from build123d import *

# Parameters (mm, degrees)
SKETCH090_R             = 5
SKETCH090_R_2           = 2.25
PAD032_DEPTH            = 2
SKETCH091_R             = 5
SKETCH091_R_2           = 3.75
PAD033_DEPTH            = 4
BODY011_PLACEMENT_ANGLE = 90


with BuildPart() as part:
    # Sketch090 → Pad032 (new body)
    with BuildSketch(Plane.XZ):
        Circle(SKETCH090_R)
        Circle(SKETCH090_R_2, mode=Mode.SUBTRACT)
    extrude(amount=PAD032_DEPTH)

    # Sketch091 (on Face4 of Pad032) → Pad033 (join)
    with BuildSketch(Plane.XZ.offset(2)):
        Circle(SKETCH091_R)
        Circle(SKETCH091_R_2, mode=Mode.SUBTRACT)
    extrude(amount=PAD033_DEPTH)


with BuildPart() as part_1:
    # Body011 placement: moved
    add(part.part.moved(Location((62, 89, 34))).rotate(Axis((62, 89, 34), (-1, 0, 0)), BODY011_PLACEMENT_ANGLE))


solid = part_1.part
Source: CAD feature listing. Evaluate the final solid. Frame: model axes, mm. A direction names the side the tool comes from. Round coordinates to 2 decimals unless told otherwise and drop trailing zeros. Loops run counter-clockwise (first coordinate to the right, second up) from the corner with the lowest first, then second, coordinate; pieces in that order, holes last.
Q1. First-contact query: P1, Ø2, axis at y = 87, z = 38.5, coming from the +X side; P2, Ø3, axis at x = 65, z = 36.5, coming from the -Y side; P3, Ø1, axis at y = 90, z = 37, coming from the +X side. Flat tips, straight axial feed; report the tip coordinate or a pass-through.
Q2. Section C-C, the plane y = 92. Return loops of the section in (x, z).
Q3. Mould query, pull axis Y, two halves, no side actions, for faces 3 (the face through (63, 93, 40)), 4 (the face through (60.92, 84.12, 36.96)), 5 (the face through (64, 87, 36)). Classes: pulls with the +Y half, pulls with the -Y half, needs draft (parallel to the pull), parting line crosses it, or undercut.
Q4. Access query for faces 1 (the face through (64.2, 88, 34)), 2 (the face through (64.02, 92.16, 37.97)). Directions: +Z, -Z, +X, -X, +Y, -Y. A direction counts if a zero-diameter tool reaches every point of the face in a straight line with its end or side. Return the directions, or none.
Q5. Section A-A, the plane x = 62. Return loops of the section in (y, z).
Q6. Section D-D, the plane z = 37.9. Return loops of the section in (x, y), plus the area to 3 significant figures.
Q7. Ray query, line 1 (Y direction, x = 62, z = 34.6); line 2 (Z direction, x = 59, y = 90.75); line 3 (X direction, y = 89.75, z = 38.7). Return the intervals inside material, ascending.
Q8. Section B-B, the plane y = 89. Return loops of the section in (x, z).
Solutions:
1. P1: stops at x = 66.9
1. P2: stops at y = 84.23
1. P3: stops at x = 66.97
2. outline: (58, 34) - (66, 34) - (66, 40) - (64.25, 40) - (64.25, 36) - (59.75, 36) - (59.75, 40) - (58, 40) - close
3. face 3: needs draft
3. face 4: parting line crosses it
3. face 5: undercut
4. face 1: -Z, +X, -X, +Y, -Y
4. face 2: +Z
5. outline: (84, 34) - (86.75, 34) - (86.75, 36) - (85.25, 36) - (85.25, 40) - (84, 40) - close; (91.25, 34) - (94, 34) - (94, 40) - (92.75, 40) - (92.75, 36) - (91.25, 36) - close
6. outline: circle Ø10 at (62, 89); hole circle Ø7.5 at (62, 89)
6. area: 34.4 mm2
7. line 1: y = 84 to 86.75, 91.25 to 94
7. line 2: z = 34 to 36
7. line 3: x = 57.06 to 58.33, 65.67 to 66.94
8. outline: (57, 34) - (59.75, 34) - (59.75, 36) - (58.25, 36) - (58.25, 40) - (57, 40) - close; (64.25, 34) - (67, 34) - (67, 40) - (65.75, 40) - (65.75, 36) - (64.25, 36) - close
